Design review of the part built by this model. Coordinates are the model's own, in mm. Round coordinates to 2 decimals unless told otherwise and drop trailing zeros. Loops run counter-clockwise (first coordinate to the right, second up) from the corner with the lowest first, then second, coordinate; pieces in that order, holes last. Notation, with made-up numbers: (-25, 65.5) - (12, 65.5) arc R26 ccw to (12, 93.5) - close; hole circle Ø3 at (64, -12). An arc over 180 degrees is marked (long way). Return JSON: item names as keys, results as strings. Group by question number.
(1) We need section C-C, the plane x = 18. Write out the cut boundary in (y, z).
(2) Clearance check with flat-ended pins moving along their axes: pin 1 (3 mm diameter, centred on x = -20.5, y = 18, fed in from +Z); pin 2 (1.5 mm diameter, centred on x = 18, z = 2, fed in from +Y). State where each tip first meets the part, or that it passes through.
(3) We need section B-B, the plane y = 0. Write out the cut boundary in (x, z).
(4) We need section D-D, the plane z = 0.5. Write out the cut boundary in (x, y), and give its area (3 significant figures).
(5) We need section A-A, the plane x = 10.5. Write out the cut boundary in (y, z).
(6) Wall thickness on L1, parallel to X at y = -20, z = 2; L2, parallel to X at y = 3.5, z = 2.2; L3, parallel to Y at x = -18, z = 0.4: over which ranges is each line inside the solid? List them lowest first. Write a range as [from, to].
from build123d import *

# Parameters (mm, degrees)
SCHIZZO1_W                   = 61.1
SCHIZZO1_H                   = 20
SCHIZZO1_R                   = 6.5
SCHIZZO1_W_2                 = 19.2
SCHIZZO1_H_2                 = 12.4
ESTRUSIONE_ESTRUSIONE1_DEPTH = 3
SCHIZZO5_W                   = 61.1
SCHIZZO5_H                   = 20
ESTRUSIONE_ESTRUSIONE2_DEPTH = 3
SCHIZZO6_R                   = 2.7
TAGLIO_ESTRUSIONE1_DEPTH     = 3
SCHIZZO7_R                   = 5
TAGLIO_ESTRUSIONE2_DEPTH     = 1.6
SMUSSO1_SIZE                 = 2


with BuildPart() as part:
    # Schizzo1 → Estrusione-Estrusione1 (new body)
    with BuildSketch(Plane.XY):
        Rectangle(SCHIZZO1_W, SCHIZZO1_H)
        with Locations((-16.55, 0)):
            Circle(SCHIZZO1_R, mode=Mode.SUBTRACT)
        with Locations((13.45, 0)):
            Rectangle(SCHIZZO1_W_2, SCHIZZO1_H_2, mode=Mode.SUBTRACT)
    extrude(amount=ESTRUSIONE_ESTRUSIONE1_DEPTH)

    # Schizzo5 → Estrusione-Estrusione2 (add)
    with BuildSketch(Plane.XY.offset(3)):
        with Locations((0, 20)):
            Rectangle(SCHIZZO5_W, SCHIZZO5_H)
    estrusione_estrusione2 = extrude(amount=-ESTRUSIONE_ESTRUSIONE2_DEPTH)

    # Schizzo6 → Taglio-Estrusione1 (cut)
    with BuildSketch(Plane.XY.offset(3)):
        with Locations((-18, 20)):
            Circle(SCHIZZO6_R)
        with Locations((18, 20)):
            Circle(SCHIZZO6_R)
    taglio_estrusione1 = extrude(amount=-TAGLIO_ESTRUSIONE1_DEPTH, mode=Mode.SUBTRACT)

    # Schizzo7 → Taglio-Estrusione2 (cut)
    with BuildSketch(Plane.XY.offset(3)):
        with Locations((-18, 20)):
            Circle(SCHIZZO7_R)
        with Locations((18, 20)):
            Circle(SCHIZZO7_R)
    taglio_estrusione2 = extrude(amount=-TAGLIO_ESTRUSIONE2_DEPTH, mode=Mode.SUBTRACT)

    # Specchia2: Estrusione-Estrusione2, Taglio-Estrusione1, Taglio-Estrusione2 across plane
    add(estrusione_estrusione2.mirror(Plane.ZX))
    add(taglio_estrusione1.mirror(Plane.ZX), mode=Mode.SUBTRACT)
    add(taglio_estrusione2.mirror(Plane.ZX), mode=Mode.SUBTRACT)

    # Smusso1
    smusso1_edges = [part.edges().sort_by_distance(p)[0] for p in [
        (0, 30, 3),
        (0, -30, 3),
    ]]
    chamfer(smusso1_edges, length=SMUSSO1_SIZE)


solid = part.part
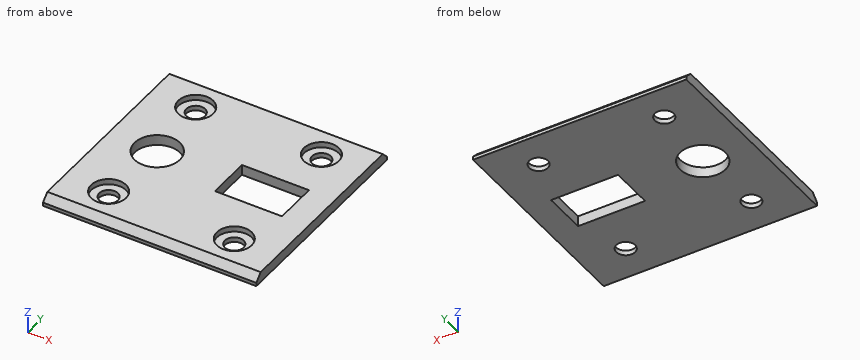
Solutions:
{
 "1": {"outline": "(-30, 0) - (-22.7, 0) - (-22.7, 1.4) - (-25, 1.4) - (-25, 3) - (-28, 3) - (-30, 1) - close; (-17.3, 0) - (-6.2, 0) - (-6.2, 3) - (-15, 3) - (-15, 1.4) - (-17.3, 1.4) - close; (6.2, 0) - (17.3, 0) - (17.3, 1.4) - (15, 1.4) - (15, 3) - (6.2, 3) - close; (22.7, 0) - (30, 0) - (30, 1) - (28, 3) - (25, 3) - (25, 1.4) - (22.7, 1.4) - close"},
 "2": {"pin 1": "z = 1.4", "pin 2": "y = 29.75"},
 "3": {"outline": "(-30.55, 0) - (-23.05, 0) - (-23.05, 3) - (-30.55, 3) - close; (-10.05, 0) - (3.85, 0) - (3.85, 3) - (-10.05, 3) - close; (23.05, 0) - (30.55, 0) - (30.55, 3) - (23.05, 3) - close"},
 "4": {"outline": "(-30.55, -30) - (30.55, -30) - (30.55, 30) - (-30.55, 30) - close; hole circle Ø13 at (-16.55, 0); hole circle Ø5.4 at (-18, -20); hole circle Ø5.4 at (-18, 20); hole (3.85, -6.2) - (23.05, -6.2) - (23.05, 6.2) - (3.85, 6.2) - close; hole circle Ø5.4 at (18, -20); hole circle Ø5.4 at (18, 20)", "area": "3,200 mm^2"},
 "5": {"outline": "(-30, 0) - (-6.2, 0) - (-6.2, 3) - (-28, 3) - (-30, 1) - close; (6.2, 0) - (30, 0) - (30, 1) - (28, 3) - (6.2, 3) - close"},
 "6": {"L1": "[-30.55, -23], [-13, 13], [23, 30.55]", "L2": "[-30.55, -22.03], [-11.07, 3.85], [23.05, 30.55]", "L3": "[-30, -22.7], [-17.3, -6.34], [6.34, 17.3], [22.7, 30]"}
}
